The model under review builds one solid part; all positions refer to its coordinate system, in mm. A direction names the side the tool comes from. Coordinates: 2 decimals unless noted, no trailing zeros. Write each loop counter-clockwise with the first axis right and the second up, starting at its lowest first coordinate (ties: lowest second). Pieces come first, ordered by that corner, then holes. Notation, with made-up numbers: M 9,-37 L 39,-37 A5 cw 39,-33 Z; hole C 7.25,-25.5 d1. An arc over 180 degrees is marked long. Answer as CSV lines item,"result". Start each with the question number.
from build123d import *

# Parameters (mm, degrees)
SKETCH_2_W          = 67
SKETCH_2_H          = 40
EXTRUDE_1_DEPTH     = 3
OTHER_START         = -15.645963378
OTHER_1_DEPTH       = 40
OTHER_1_2_DEPTH     = 40
SKETCH_8_W          = 5
SKETCH_8_H          = 30
EXTRUDE_2_DEPTH     = 18
FILLET_2_R          = 15
FILLET_3_R          = 15
SKETCH_9_R          = 2.44
CUT_EXTRUDE_1_DEPTH = 43


# Read off the part's stored shape, not the designer's step: 绘制的折弯1
with BuildPart() as part:
    # Sketch 2 → 凸台-拉伸1 (new body)
    with BuildSketch(Plane.XY):
        with Locations((-0.762466526, 4.354036622)):
            Rectangle(SKETCH_2_W, SKETCH_2_H)
    extrude(amount=EXTRUDE_1_DEPTH)

    # Other 1 outline → Other 1 (cut)
    with BuildSketch(Plane(origin=(0, 0, 0), x_dir=(1, 0, 0), z_dir=(0, 1, 0)).offset(OTHER_START)):
        with BuildLine():
            Line((-34.262466526, -3), (-17.135449872, -3))
            ThreePointArc((-17.135449872, -3), (-15.711956269, -0.83772234), (-13.262466526, 0))
            Line((-13.262466526, 0), (-34.262466526, 0))
            Line((-34.262466526, 0), (-34.262466526, -3))
        make_face()
        with BuildLine():
            ThreePointArc((11.737533474, 0), (14.187023217, -0.83772234), (15.61051682, -3))
            Line((15.61051682, -3), (32.737533474, -3))
            Line((32.737533474, -3), (32.737533474, 0))
            Line((32.737533474, 0), (11.737533474, 0))
        make_face()
    extrude(amount=OTHER_1_DEPTH, mode=Mode.SUBTRACT)

    # Other 1 2 outline → Other 1 2 (add)
    with BuildSketch(Plane(origin=(0, 0, 0), x_dir=(1, 0, 0), z_dir=(0, 1, 0)).offset(OTHER_START)):
        with BuildLine():
            Line((-14.262466526, -21.073009183), (-14.262466526, -4))
            ThreePointArc((-14.262466526, -4), (-13.969573307, -3.292893219), (-13.262466526, -3))
            Line((-13.262466526, -3), (-17.135449872, -3))
            ThreePointArc((-17.135449872, -3), (-17.230585311, -3.49598283), (-17.262466526, -4))
            Line((-17.262466526, -4), (-17.262466526, -21.073009183))
            Line((-17.262466526, -21.073009183), (-14.262466526, -21.073009183))
        make_face()
        with BuildLine():
            Line((15.61051682, -3), (11.737533474, -3))
            ThreePointArc((11.737533474, -3), (12.444640255, -3.292893219), (12.737533474, -4))
            Line((12.737533474, -4), (12.737533474, -21.073009183))
            Line((12.737533474, -21.073009183), (15.737533474, -21.073009183))
            Line((15.737533474, -21.073009183), (15.737533474, -4))
            ThreePointArc((15.737533474, -4), (15.705652259, -3.49598283), (15.61051682, -3))
        make_face()
    extrude(amount=OTHER_1_2_DEPTH)

    # 草图8 → 凸台-拉伸2 (add)
    with BuildSketch(Plane.XY.offset(3)):
        with Locations((-0.762466526, 4.354036622)):
            Rectangle(SKETCH_8_W, SKETCH_8_H)
    extrude(amount=EXTRUDE_2_DEPTH)

    # 圆角2
    fillet_2_edges = [part.edges().sort_by_distance(p)[0] for p in [
        (-15.762466526, 24.354036622, 21.073009183),
    ]]
    fillet(fillet_2_edges, radius=FILLET_2_R)

    # 圆角3
    fillet_3_edges = [part.edges().sort_by_distance(p)[0] for p in [
        (14.237533474, -15.645963378, 21.073009183),
        (14.237533474, 24.354036622, 21.073009183),
        (-0.762466526, 19.354036622, 21),
        (-0.762466526, -10.645963378, 21),
        (-15.762466526, -15.645963378, 21.073009183),
    ]]
    fillet(fillet_3_edges, radius=FILLET_3_R - 0.0001)  # a hair under: the kernel refuses the full size

    # 草图9 → 切除-拉伸1 (cut)
    with BuildSketch(Plane(origin=(15.737533474, 0, 0), x_dir=(0, 0, -1), z_dir=(1, 0, 0))):
        with Locations(Location((-14, 4.354036622, 0), (0, 0, 90))):
            Circle(SKETCH_9_R)
    extrude(amount=-CUT_EXTRUDE_1_DEPTH, mode=Mode.SUBTRACT)


solid = part.part
1) To check wall thickness, follow line 1 (X direction, y = -3.5, z = 11); line 2 (X direction, y = -13, z = 9.25); line 3 (Z direction, x = 4.5, y = 21.5). State the ranges of each line that lie inside material, in increasing order. Write a range as [from, to].
2) Mouldability with a two-part tool opening along X and no side actions: class faces 1 (the flat face through (-17.262, 4, 11)), 2 (the flat face through (-1, 5, 0)), 3 (the flat face through (-3.262, 4, 10)) as +X half, -X half, draft (parallel to the pull), parting line (faces both ways), or undercut.
3) Clearance check with flat-ended pins moving along their axes: pin 1 Ø1 at (x, z) = (11, 11) entering from -Y; pin 2 Ø3.5 at (x, z) = (-1, 5) entering from +Y; pin 3 Ø8 at (y, z) = (4.35, 14) entering from -X; pin 4 Ø0.9 at (x, z) = (-0.5, 4.5) entering from -Y. State where each tip first meets the part, or that it passes through.
4) Tool access review of faces 4 (the flat face through (-14.262, 4, 11)), 5 (the flat face through (-1, 24.354, 2)), 6 (the cylindrical face through (-0.727, 15.077, 16.489)): name each direction out of +Z, -Z, +X, -X, +Y, -Y from which nothing blocks a thin tool from reaching the whole face with its end or side.
5) Take a section at D-D on z = 13.25. Give the boundary of the cut face in (x, y), and give its area (3 significant figures).
6) Take a section at C-C on y = -13. Give the boundary of the cut face in (x, z), and give its area (3 significant figures).
7) Take a section at A-A on z = 15.75. Give the boundary of the cut face in (x, y), and give its area (3 significant figures).
Results:
1,line 1,"x = [-17.26, -14.26], [-3.26, 1.74], [12.74, 15.74]"
1,line 2,"x = [-17.26, -14.26], [12.74, 15.74]"
1,line 3,"z = [0, 3]"
2,face 1,"-X half"
2,face 2,"draft"
2,face 3,"undercut"
3,pin 1,"passes through"
3,pin 2,"stops at y = 19.35"
3,pin 3,"stops at x = -17.26"
3,pin 4,"stops at y = -10.65"
4,face 4,"+Z, +Y, -Y"
4,face 5,"+Z, -Z, +X, -X, +Y"
4,face 6,"+Z, +Y"
5,outline,"M -17.26,-13.82 L -14.26,-13.82 L -14.26,2.03 L -17.26,2.03 Z; M -17.26,6.68 L -14.26,6.68 L -14.26,22.53 L -17.26,22.53 Z; M -3.26,-8.78 L 1.74,-8.78 L 1.74,2.03 L -3.26,2.03 Z; M -3.26,6.68 L 1.74,6.68 L 1.74,17.49 L -3.26,17.49 Z; M 12.74,-13.82 L 15.74,-13.82 L 15.74,2.03 L 12.74,2.03 Z; M 12.74,6.68 L 15.74,6.68 L 15.74,22.53 L 12.74,22.53 Z"
5,area,"298 mm²"
6,outline,"M -17.26,4 A4 ccw -13.26,0 L 11.74,0 A4 ccw 15.74,4 L 15.74,14.58 L 12.74,14.58 L 12.74,4 A1 cw 11.74,3 L -13.26,3 A1 cw -14.26,4 L -14.26,14.58 L -17.26,14.58 Z"
6,area,"162 mm²"
7,outline,"M -17.26,-12.11 L -14.26,-12.11 L -14.26,2.65 L -17.26,2.65 Z; M -17.26,6.05 L -14.26,6.05 L -14.26,20.82 L -17.26,20.82 Z; M -3.26,-7.05 L 1.74,-7.05 L 1.74,2.65 L -3.26,2.65 Z; M -3.26,6.05 L 1.74,6.05 L 1.74,15.75 L -3.26,15.75 Z; M 12.74,-12.11 L 15.74,-12.11 L 15.74,2.65 L 12.74,2.65 Z; M 12.74,6.05 L 15.74,6.05 L 15.74,20.82 L 12.74,20.82 Z"
7,area,"274 mm²"
